Check sheet for the modelled part. Datum: model origin and axes. Units: mm. Face numbers are marked on the shaded views. A direction names the side the tool comes from. Give positions to 0.01 mm unless a question says otherwise; leave off trailing zeros. Write each loop counter-clockwise with the first axis right and the second up, starting at its lowest first coordinate (ties: lowest second). Pieces come first, ordered by that corner, then holes. Notation, with made-up numbers: (41, 24.5) - (69, 24.5) arc R30 ccw to (69, 57.5) - close; hole circle Ø11 at (57.25, 84.5). An arc over 180 degrees is marked (long way). Return JSON: item names as keys, results as strings. Group by question number.
```python
from build123d import *

# Parameters (mm, degrees)
HEX_DIE_START = -2e-06
SKETCH2_R     = 8.3242194
HEX_DIE_DEPTH = 7.493002
SKETCH3_W     = 16.483602772
SKETCH3_H     = 2.3876
SLOT_DEPTH    = 4.2672
SKETCH4_R     = 6.245225
INDENT_DEPTH  = 0.936625


with BuildPart() as part:
    # BodySke → Base-Revolve (revolve)
    with BuildSketch(Plane.XY, mode=Mode.PRIVATE) as base_revolve_sk:
        Polygon((7.493, 4.7625), (7.493, 8.241801386), (0.637626437, 8.241801386), (0, 7.1374), (0, 0), (45.593, 0), (45.593, 4.7625), align=None)
    revolve(base_revolve_sk.sketch.rotate(Axis((-25.4, 0, 0), (1, 0, 0)), 90), axis=Axis((-25.4, 0, 0), (1, 0, 0)))

    # Sketch2 → Hex-Die (cut)
    with BuildSketch(Plane(origin=(0, 0, 0), x_dir=(0, 0, -1), z_dir=(1, 0, 0)).offset(HEX_DIE_START)):
        Circle(SKETCH2_R)
        Polygon((-7.1374, 4.120779829), (0, 8.241559659), (7.1374, 4.120779829), (7.1374, -4.120779829), (0, -8.241559659), (-7.1374, -4.120779829), align=None, mode=Mode.SUBTRACT)
    extrude(amount=HEX_DIE_DEPTH, mode=Mode.SUBTRACT)

    # Sketch3 → Slot (cut)
    with BuildSketch(Plane(origin=(0, 0, 0), x_dir=(0, 0, -1), z_dir=(1, 0, 0))):
        Rectangle(SKETCH3_W, SKETCH3_H)
    extrude(amount=SLOT_DEPTH, mode=Mode.SUBTRACT)

    # Sketch4 → Indent (cut)
    with BuildSketch(Plane(origin=(0, 0, 0), x_dir=(0, 0, -1), z_dir=(1, 0, 0))):
        Circle(SKETCH4_R)
    extrude(amount=INDENT_DEPTH, mode=Mode.SUBTRACT)


solid = part.part
```
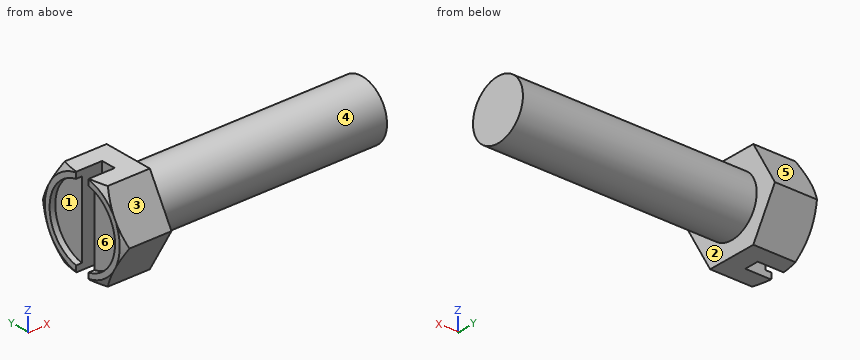
Item 1: Mould release check, pull along Z, two halves, no side actions. Record for the marked faces 1, 2, 3 and 4: +Z half, -Z half, draft (parallel to the pull), parting line (faces both ways), or undercut.
Item 2: Material ranges on line 1 along X through (y, z) = (-5.25, -3.5); line 2 along X through (y, z) = (0, 5); line 3 along Z through (x, y) = (15.5, 1.5), recorded low to high. Write a range as from..to.
Item 3: Section check A-A on x = 28. Record the cut outline in (y, z) (1 decimal).
Item 4: Access from +Z, -Z, +X, -X, +Y, -Y to the whole of each face (thin tool, end or side, straight path). Record for the marked faces 5 and 6.
Item 5: Depth check by flat-ended pin: pin 1 (1 mm diameter, centred on x = 33, z = 4.5, fed in from -Y); pin 2 (1.5 mm diameter, centred on y = 2.5, z = 1.5, fed in from -X); pin 3 (8 mm diameter, centred on x = 17.5, y = 0.5, fed in from -Z). Enter the tip coordinate at first touch or a pass-through.
Reply:
{
 "1": {"face 1": "undercut", "face 2": "draft", "face 3": "+Z half", "face 4": "parting line"},
 "2": {"line 1": "0..7.49", "line 2": "4.27..7.49", "line 3": "-4.52..4.52"},
 "3": {"outline": "circle Ø9.5 at (0, 0)"},
 "4": {"face 5": "+Z, +X, -X, +Y", "face 6": "-X"},
 "5": {"pin 1": "y = -2.58", "pin 2": "x = 0.94", "pin 3": "z = -4.76"}
}
